The listing builds one solid part. Answer for the finished solid, in the listing's coordinates (mm). Face numbers are marked on the shaded views. A direction names the side the tool comes from. Give positions to 0.01 mm unless a question says otherwise; leave off trailing zeros. Order: outer loops, then holes, each group sorted by start corner. A loop starts at its lowest first (then second) coordinate and runs counter-clockwise, first axis right, second up. Notation, with made-up numbers: (24.5, -9.5) - (53.5, -9.5) arc R21 cw to (53.5, 4.5) - close; hole circle Ø5 at (65.25, 24.5). An arc over 180 degrees is marked (long way). Write each question's results on one line, items separated by ' | '. Start each with the question number.
1. Section C-C (z = -18.5) is taken. Give the vertices of the cut face in (x, y), and give its area (3 significant figures).
2. Section D-D (y = 25) is taken. Give the vertices of the cut face in (x, z).
3. Section A-A (x = 20.5) is taken. Give the vertices of the cut face in (y, z), and give its area (3 significant figures).
4. Section B-B (y = 19) is taken. Give the vertices of the cut face in (x, z), and give its area (3 significant figures).
5. Which of the six approach directions +Z, -Z, +X, -X, +Y, -Y give full straight-line access (tool end or side, diameter ignored) to the marked faces 1 and 2?
6. Flat-ended cylindrical pins translate along their axes: pin 1 (1 mm diameter, centred on x = -0.5, y = 13.5, fed in from -Z); pin 2 (2.5 mm diameter, centred on y = 24, z = -3.08, fed in from -X); pin 3 (6 mm diameter, centred on x = 12.5, z = -13.5, fed in from +Y); pin 4 (11 mm diameter, centred on y = 18.5, z = -23.5, fed in from +X). Find the tip coordinate at first contact, or state that the pin passes through.
7. Find the intervals of material crossed by L1, parallel to X at y = 0.9, z = -3.25; L2, parallel to X at y = 25, z = -32; L3, parallel to Y at x = 31.5, z = -29.5, in increasing order.
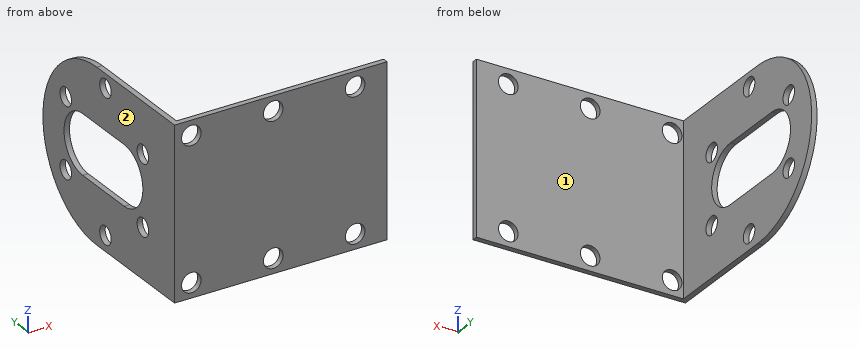
from build123d import *

# Parameters (mm, degrees)
ESQUISSE1_W             = 45.5
ESQUISSE1_H             = 37.5
ESQUISSE1_R             = 2.15
BOSS_EXTRU_1_DEPTH      = 1.2
BOSS_EXTRU_2_DEPTH      = 1.2
ENL_V_MAT_EXTRU_2_DEPTH = 75.623947588
ESQUISSE9_R             = 2
ENL_V_MAT_EXTRU_3_DEPTH = 75.623947588


with BuildPart() as part:
    # Esquisse1 → Boss.-Extru.1 (new body)
    with BuildSketch(Plane(origin=(0, 0, 0), x_dir=(1, 0, 0), z_dir=(0, 1, 0))):
        with Locations((22.75, 18.75)):
            Rectangle(ESQUISSE1_W, ESQUISSE1_H)
        with Locations(Location((2.5, 34.25, 0), (0, 0, 270))):
            Circle(ESQUISSE1_R, mode=Mode.SUBTRACT)
        with Locations(Location((20.5, 34.25, 0), (0, 0, 270))):
            Circle(ESQUISSE1_R, mode=Mode.SUBTRACT)
        with Locations(Location((38.5, 34.25, 0), (0, 0, 270))):
            Circle(ESQUISSE1_R, mode=Mode.SUBTRACT)
        with Locations(Location((2.5, 3.25, 0), (0, 0, 270))):
            Circle(ESQUISSE1_R, mode=Mode.SUBTRACT)
        with Locations(Location((20.5, 3.25, 0), (0, 0, 270))):
            Circle(ESQUISSE1_R, mode=Mode.SUBTRACT)
        with Locations(Location((38.5, 3.25, 0), (0, 0, 270))):
            Circle(ESQUISSE1_R, mode=Mode.SUBTRACT)
    extrude(amount=BOSS_EXTRU_1_DEPTH)

    # Esquisse4 → Boss.-Extru.2 (add)
    with BuildSketch(Plane.ZY):
        with BuildLine():
            Line((-37.48187916, 0), (-37.48187916, 27))
            ThreePointArc((-37.48187916, 27), (-18.74093958, 45.74093958), (0, 27))
            Line((0, 27), (0, 0))
            Line((0, 0), (-37.48187916, 0))
        make_face()
    extrude(amount=BOSS_EXTRU_2_DEPTH)

    # Esquisse5 → Enlèv. mat.-Extru.2 (cut, through all)
    with BuildSketch(Plane(origin=(0, 0, 0), x_dir=(0, 0, -1), z_dir=(1, 0, 0))):
        with BuildLine():
            Line((25, 31.9), (25, 17.5))
            ThreePointArc((25, 17.5), (18.5, 11), (12, 17.5))
            Line((12, 17.5), (12, 31.9))
            ThreePointArc((12, 31.9), (18.5, 38.4), (25, 31.9))
        make_face()
    extrude(amount=-ENL_V_MAT_EXTRU_2_DEPTH, mode=Mode.SUBTRACT)

    # Esquisse9 → Enlèv. mat.-Extru.3 (cut, through all)
    with BuildSketch(Plane(origin=(0, 0, 0), x_dir=(0, 0, -1), z_dir=(1, 0, 0))):
        with Locations((26.48187916, 11)):
            Circle(ESQUISSE9_R)
        with Locations((26.48187916, 37.8)):
            Circle(ESQUISSE9_R)
        with Locations((11.08187916, 11)):
            Circle(ESQUISSE9_R)
        with Locations((11.08187916, 37.8)):
            Circle(ESQUISSE9_R)
        with Locations((34.08187916, 24)):
            Circle(ESQUISSE9_R)
        with Locations((3.08187916, 24)):
            Circle(ESQUISSE9_R)
    extrude(amount=-ENL_V_MAT_EXTRU_3_DEPTH, mode=Mode.SUBTRACT)


solid = part.part
Reported:
1) outline: (-1.2, 0) - (45.5, 0) - (45.5, 1.2) - (0, 1.2) - (0, 11) - (-1.2, 11) - close; (-1.2, 38.4) - (0, 38.4) - (0, 45.74) - (-1.2, 45.74) - close | area: 76.6 mm²
2) outline: (-1.2, -37.48) - (0, -37.48) - (0, -35.81) - (-1.2, -35.81) - close; (-1.2, -32.35) - (0, -32.35) - (0, -25) - (-1.2, -25) - close; (-1.2, -12) - (0, -12) - (0, -4.81) - (-1.2, -4.81) - close; (-1.2, -1.35) - (0, -1.35) - (0, 0) - (-1.2, 0) - close
3) outline: (0, -37.5) - (1.2, -37.5) - (1.2, -36.4) - (0, -36.4) - close; (0, -32.1) - (1.2, -32.1) - (1.2, -5.4) - (0, -5.4) - close; (0, -1.1) - (1.2, -1.1) - (1.2, 0) - (0, 0) - close | area: 34.7 mm²
4) outline: (-1.2, -37.48) - (0, -37.48) - (0, -25) - (-1.2, -25) - close; (-1.2, -12) - (0, -12) - (0, 0) - (-1.2, 0) - close | area: 29.4 mm²
5) face 1: +Z, -Z, +X, +Y | face 2: +Z, -Z, -X, +Y, -Y
6) pin 1: z = -37.48 | pin 2: through | pin 3: y = 1.2 | pin 4: x = 0
7) L1: -1.2 to 0.35, 4.65 to 18.35, 22.65 to 36.35, 40.65 to 45.5 | L2: -1.2 to 0 | L3: 0 to 1.2
